The listing builds one solid part. Answer for the finished solid, in the listing's coordinates (mm). Give positions to 0.01 mm unless a question says otherwise; leave off trailing zeros. Loops run counter-clockwise (first coordinate to the right, second up) from the corner with the lowest first, then second, coordinate; pieces in that order, holes last. Notation, with made-up numbers: M 84,74.25 L 130,74.25 A33 cw 130,103.25 Z; hole C 49,59.5 d9. An arc over 180 degrees is marked long. Return JSON: item names as keys, results as strings.
from build123d import *

# Parameters (mm, degrees)
F0_R     = 11.1
F1_DEPTH = 7
F2_SIZE2 = 0.5
F2_SIZE  = 1.5
F3_R     = 2


with BuildPart() as f1:
    # F0 (on Top) → F1 (new body)
    with BuildSketch(Plane.XY):
        with BuildLine():
            ThreePointArc((-31.251265, 9.347386), (-28, 0), (-31.251265, -9.347386))
            ThreePointArc((-31.251265, -9.347386), (-14, -45), (3.251265, -9.347386))
            ThreePointArc((3.251265, -9.347386), (0, 0), (3.251265, 9.347386))
            ThreePointArc((3.251265, 9.347386), (-14, 45), (-31.251265, 9.347386))
        make_face()
        with Locations((-14, 0)):
            Circle(F0_R, mode=Mode.SUBTRACT)
    extrude(amount=F1_DEPTH)

    # F2
    f2_edges = [f1.edges().sort_by_distance(p)[0] for p in [
        (-25.1, 0, 7),
        (-25.1, 0, 0),
    ]]
    chamfer(f2_edges, length=F2_SIZE, length2=F2_SIZE2)

    # F3
    f3_edges = [f1.edges().sort_by_distance(p)[0] for p in [
        (-14, -45, 7),
        (-14, -45, 0),
    ]]
    fillet(f3_edges, radius=F3_R)


solid = f1.part
(1) The part is cut by section C-C (z = 4). Determine the outline of the cut face in (x, y) (1 decimal), and give its area (3 significant figures).
Values follow:
{"outline": "M -31.3,-9.3 A22 ccw long 3.3,-9.3 A15.1 cw 3.3,9.3 A22 ccw long -31.3,9.3 A15.1 cw Z; hole C -14,0 d22.2", "area": "2,810 mm²"}
(2) The part is cut by section A-A (y = 0). Determine the outline of the cut face in (x, z), and give its area (3 significant figures).
Values follow:
{"outline": "M -28,2 A2 ccw -26,0 L -25.6,0 L -25.1,1.5 L -25.1,5.5 L -25.6,7 L -26,7 A2 ccw -28,5 Z; M -2.9,1.5 L -2.4,0 L -2,0 A2 ccw 0,2 L 0,5 A2 ccw -2,7 L -2.4,7 L -2.9,5.5 Z", "area": "35.7 mm²"}
(3) Determine the mould class of faces 1 (the cylindrical face through (-3.4, 3.3, 3.5)), 2 (the cylindrical face through (-13.31, 44.99, 3.48)), 3 (the flat face through (-5, -9, 7)) for opening direction X: released by +X, released by -X, zero draft, split by the parting line, or undercut.
Values follow:
{"face 1": "undercut", "face 2": "split by the parting line", "face 3": "zero draft"}
(4) The part is cut by section B-B (x = -14). Determine the outline of the cut face in (y, z), and give its area (3 significant figures).
Values follow:
{"outline": "M -45,2 A2 ccw -43,0 L -11.6,0 L -11.1,1.5 L -11.1,5.5 L -11.6,7 L -43,7 A2 ccw -45,5 Z; M 11.1,1.5 L 11.6,0 L 43,0 A2 ccw 45,2 L 45,5 A2 ccw 43,7 L 11.6,7 L 11.1,5.5 Z", "area": "470 mm²"}
(5) Straight lines are drawn through the part: line 1 along Y through (x, z) = (-14.5, 3.75); line 2 along Y through (x, z) = (-10.5, 6.5); line 3 along X through (y, z) = (3, 1.75). For each, find the intervals that lie inside material, in ascending order.
Values follow:
{"line 1": "-44.99 to -11.09, 11.09 to 44.99", "line 2": "-44.03 to -10.88, 10.88 to 44.03", "line 3": "-28.29 to -24.69, -3.31 to 0.29"}
(6) Given pin 1 (13.5 mm diameter, centred on x = -14, y = 0, fed in from -Z); pin 2 (2 mm diameter, centred on x = -28.5, z = 6, fed in from +Y); pin 3 (3 mm diameter, centred on y = 11.5, z = 2.5, fed in from +X); pin 4 (1 mm diameter, centred on x = -8, y = 13, fed in from -Z), each flat-ended and moving along its own axis, determine where each tip first touches the part or whether it passes through.
Values follow:
{"pin 1": "through", "pin 2": "y = 40.19", "pin 3": "x = 5.6", "pin 4": "z = 0"}
